Design review of the part shown in the three views and the two pictorial views. Dimensions are in mm from the part's minimum x, y and z. A direction names the side the tool comes from. Round coordinates to 2 decimals unless told otherwise and drop trailing zeros. Order: outer loops, then holes, each group sorted by start corner. A loop starts at its lowest first (then second) coordinate and runs counter-clockwise, first axis right, second up. Notation, with made-up numbers: M 89,-38 L 106,-38 A20 cw 106,-8 Z; hole C 9.25,46.25 d5. An arc over 180 degrees is marked long. Write each question's results on one line, items separated by ' | '. Start each with the question number.
Item 1: Clearance check with flat-ended pins moving along their axes: pin 1 (2 mm diameter, centred on y = 179, z = 134, fed in from +X); pin 2 (14.5 mm diameter, centred on x = 234.5, z = 117, fed in from +Y). State where each tip first meets the part, or that it passes through.
Item 2: Take a section at A-A, the plane z = 104.5. Write out the cut boundary in (x, y), plus the area to 3 significant figures.
Item 3: Machinability: for the marked faces 1, 2 and 3, which of the approach directions +Z, -Z, +X, -X, +Y, -Y give a long, thin tool a straight path to every point of the face, cutting with its end or side? Answer none if there is none.
Item 4: Wall thickness on line 1 (X direction, y = 202, z = 40); line 2 (Z direction, x = 211, y = 96): over which ranges is each line inside the solid? List them lowest first. Write a range as [from, to].
Item 5: Take a section at C-C, the plane x = 224. Write out the cut boundary in (y, z).
Item 6: Take a section at B-B, the plane y = 189.5. Write out the cut boundary in (x, z), plus the area to 3 significant figures.
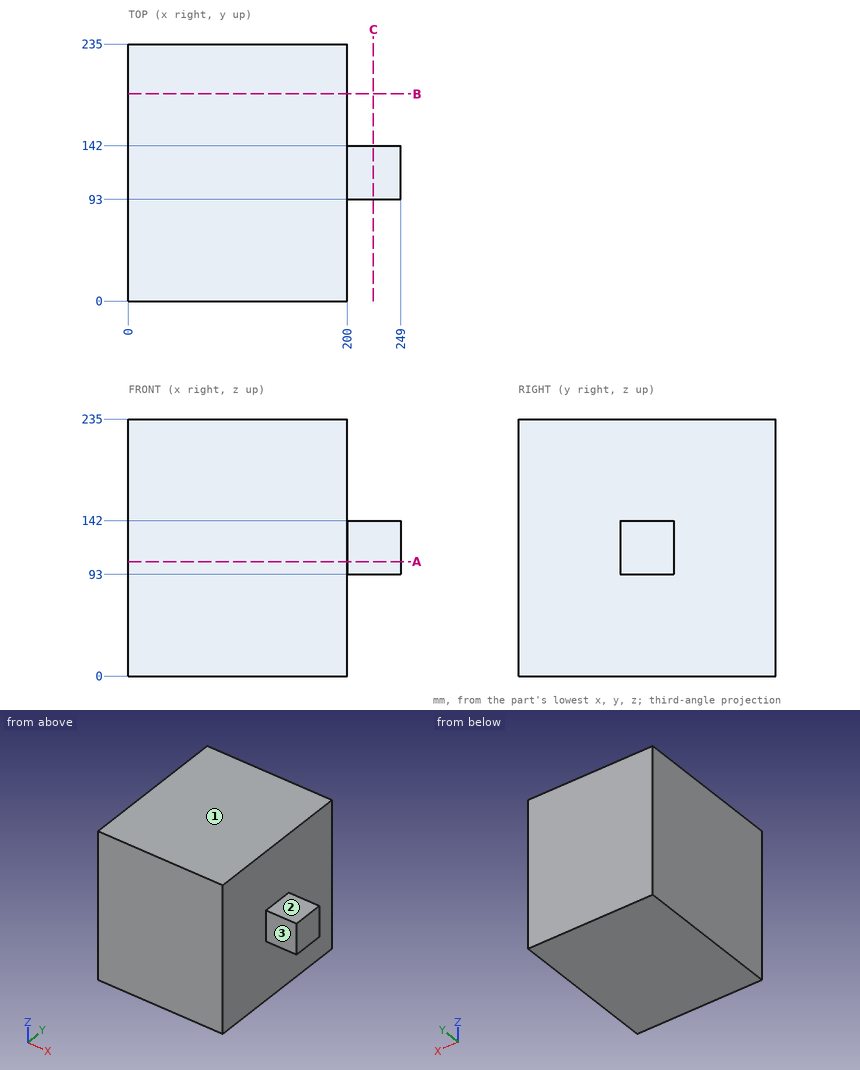
Results list:
1) pin 1: x = 200 | pin 2: y = 142
2) outline: M 0,0 L 200,0 L 200,93 L 249,93 L 249,142 L 200,142 L 200,235 L 0,235 Z | area: 49,400 mm²
3) face 1: +Z, +X, -X, +Y, -Y | face 2: +Z, +X, +Y, -Y | face 3: +Z, -Z, +X, -Y
4) line 1: [0, 200] | line 2: [93, 142]
5) outline: M 93,93 L 142,93 L 142,142 L 93,142 Z
6) outline: M 0,0 L 200,0 L 200,235 L 0,235 Z | area: 47,000 mm²
